from build123d import *

# Parameters (mm, degrees)
F1_DEPTH = 90
F2_T     = -2.5
F4_DEPTH = 90.001


with BuildPart() as f1:
    # F0 (on Front) → F1 (new body)
    with BuildSketch(Plane.XZ):
        with BuildLine():
            ThreePointArc((-27.5, 0), (0, -27.5), (27.5, 0))
            ThreePointArc((27.5, 0), (0, 27.5), (-27.5, 0))
        make_face()
        with BuildLine():
            Line((27.5, -36), (27.5, 0))
            ThreePointArc((27.5, 0), (0, -27.5), (-27.5, 0))
            Line((-27.5, 0), (-27.5, -36))
            Line((-27.5, -36), (27.5, -36))
        make_face()
    extrude(amount=-F1_DEPTH)

    # F2
    f2_openings = [f1.faces().sort_by_distance(p)[0] for p in [
        (0, 0, -6.873738),
        (0, 45, -36),
    ]]
    offset(amount=F2_T, openings=f2_openings)

    # F3 (on face) → F4 (cut, through all)
    with BuildSketch(Plane(origin=(0, 90, 0), x_dir=(-1, 0, 0), z_dir=(0, 1, 0))):
        with BuildLine():
            ThreePointArc((5, -16), (0, -11), (-5, -16))
            Line((-5, -16), (-5, -36))
            Line((-5, -36), (5, -36))
            Line((5, -36), (5, -16))
        make_face()
    extrude(amount=-F4_DEPTH, mode=Mode.SUBTRACT)


solid = f1.part
Verification items for the finished model (mm, model axes). A direction names the side the tool comes from. Give positions to 0.01 mm unless a question says otherwise; leave off trailing zeros. Order: outer loops, then holes, each group sorted by start corner. A loop starts at its lowest first (then second) coordinate and runs counter-clockwise, first axis right, second up. Notation, with made-up numbers: M -34.5,36 L 11.5,36 A32 ccw 11.5,72 Z; hole C 29.25,-14.5 d2. An arc over 180 degrees is marked long. Answer as a JSON object with one key per item and string values. Group by question number.
1) Mould release check, pull along X, two halves, no side actions. Record for faces 1 (the face through (0, 90, -4)), 2 (the face through (-27.5, 44, -18)), 3 (the face through (0, 87.5, -5)), 4 (the face through (0.55, 43.138, 24.994)): released by +X, released by -X, zero draft, split by the parting line, or undercut.
2) Cross-section at B-B (z = -2). Enter the section's corners in (x, y).
3) Access from +Z, -Z, +X, -X, +Y, -Y to the whole of each face (thin tool, end or side, straight path). Record for faces 5 (the face through (-25, 43, -18)), 6 (the face through (-8, 0, 24)), 7 (the face through (5, 89, -26)).
4) Scan lines: line 1 along X through (y, z) = (25.5, -16); line 2 along Y through (x, z) = (4.5, -10.5); line 3 along X through (y, z) = (36.5, 3.5). Record each from-to range of solid material in increasing order. Write a range as [from, to].
5) Cross-section at C-C (y = 6.5). Enter the section's corners in (x, z).
6) Cross-section at D-D (x = 0). Enter the section's corners in (y, z), then the cut area to 3 significant figures.
7) Cross-section at A-A (z = -19). Enter the section's corners in (x, y).
8) Depth check by flat-ended pin: pin 1 Ø10 at (x, y) = (-10.5, 57) entering from -Z; pin 2 Ø6 at (x, z) = (-11.5, -24) entering from -Y; pin 3 Ø4 at (x, y) = (11.5, 10) entering from +Z. Enter the tip coordinate at first touch or a pass-through.
Result sheet:
{
 "1": {"face 1": "zero draft", "face 2": "released by -X", "face 3": "undercut", "face 4": "undercut"},
 "2": {"outline": "M -27.5,0 L -25,0 L -25,87.5 L 25,87.5 L 25,0 L 27.5,0 L 27.5,90 L -27.5,90 Z"},
 "3": {"face 5": "-Z, -Y", "face 6": "+Z, -Z, +X, -X, -Y", "face 7": "-Z, +Y, -Y"},
 "4": {"line 1": "x = [-27.5, -25], [25, 27.5]", "line 2": "y = [87.5, 90]", "line 3": "x = [-27.28, -24.75], [24.75, 27.28]"},
 "5": {"outline": "M -27.5,-36 L -25,-36 L -25,0 A25 cw 25,0 L 25,-36 L 27.5,-36 L 27.5,0 A27.5 ccw -27.5,0 Z"},
 "6": {"outline": "M 0,25 L 87.5,25 L 87.5,-11 L 90,-11 L 90,27.5 L 0,27.5 Z", "area": "315 mm2"},
 "7": {"outline": "M -27.5,0 L -25,0 L -25,87.5 L -5,87.5 L -5,90 L -27.5,90 Z; M 5,87.5 L 25,87.5 L 25,0 L 27.5,0 L 27.5,90 L 5,90 Z"},
 "8": {"pin 1": "stops at z = 19.62", "pin 2": "stops at y = 87.5", "pin 3": "stops at z = 25.81"}
}
